Work out the finished part from the listing and answer in its coordinate system (mm). Face numbers are marked on the shaded views. Give positions to 0.01 mm unless a question says otherwise; leave off trailing zeros. Order: outer loops, then holes, each group sorted by start corner. A loop starts at its lowest first (then second) coordinate and runs counter-clockwise, first axis right, second up. Notation, with made-up numbers: (23, 86) -> (68, 86) arc R7 ccw to (68, 98) -> close; hole circle Ø7 at (28, -23). An arc over 180 degrees is marked (long way). Use a Markdown table: item, result. Add a question column.
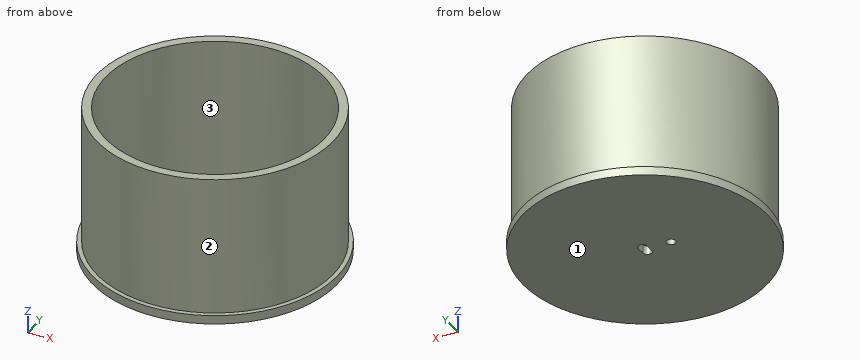
```python
from build123d import *

# Parameters (mm, degrees)
SKETCH1_R           = 88.9
BOSS_EXTRUDE1_DEPTH = 6.35
SKETCH2_R           = 3.302
CUT_EXTRUDE1_DEPTH  = 126.88384527
SKETCH3_R           = 85.725
SKETCH3_R_2         = 79.375
BOSS_EXTRUDE2_DEPTH = 101.6


with BuildPart() as part:
    # Sketch1 → Boss-Extrude1 (new body)
    with BuildSketch(Plane.XY):
        Circle(SKETCH1_R)
    extrude(amount=BOSS_EXTRUDE1_DEPTH)

    # Sketch2 → Cut-Extrude1 (cut, through all)
    with BuildSketch(Plane(origin=(0, 0, 0), x_dir=(-1, 0, 0), z_dir=(0, 0, -1))):
        with Locations((19.05, 0)):
            Circle(SKETCH2_R)
        with BuildLine():
            Line((3.081986422, 3.266652236), (3.265367316, -3.083347764))
            ThreePointArc((3.265367316, -3.083347764), (0.183342684, -6.348676869), (-3.081986422, -3.266652236))
            Line((-3.081986422, -3.266652236), (-3.265367316, 3.083347764))
            ThreePointArc((-3.265367316, 3.083347764), (-0.183342684, 6.348676869), (3.081986422, 3.266652236))
        make_face()
    extrude(amount=-CUT_EXTRUDE1_DEPTH, mode=Mode.SUBTRACT)

    # Sketch3 → Boss-Extrude2 (add)
    with BuildSketch(Plane.XY.offset(6.35)):
        Circle(SKETCH3_R)
        Circle(SKETCH3_R_2, mode=Mode.SUBTRACT)
    extrude(amount=BOSS_EXTRUDE2_DEPTH)


solid = part.part
```
1) Flat-ended cylindrical pins translate along their axes: pin 1 (10 mm diameter, centred on y = -69, z = 66.5, fed in from +X); pin 2 (1 mm diameter, centred on y = -68.5, z = 67, fed in from +X); pin 3 (10.5 mm diameter, centred on x = -19.05, y = 0, fed in from +Z). Find the tip coordinate at first contact, or state that the pin passes through.
2) The part is cut by section B-B, the plane y = 0. Determine the outline of the cut face in (x, z) (3 decimals).
3) The part is cut by section D-D, the plane y = 49. Determine the outline of the cut face in (x, z), then the cut area to 3 significant figures.
4) The part is cut by section C-C, the plane z = 86. Determine the outline of the cut face in (x, y) (3 decimals).
5) Determine the mould class of the marked faces 1, 2 and 3 for opening direction X: released by +X, released by -X, zero draft, split by the parting line, or undercut.
6) The part is cut by section A-A, the plane x = 0. Determine the outline of the cut face in (y, z) (3 decimals).
7) Straight lines are drawn through the part: line 1 (Y direction, x = 0, z = 27) (3 decimals); line 2 (Z direction, x = 72.5, y = -21); line 3 (X direction, y = 36.5, z = 52). For each, find the intervals that lie inside material, in ascending order.
A:
| question | item | result |
|---|---|---|
| 1 | pin 1 | x = 57.03 |
| 1 | pin 2 | x = 52.2 |
| 1 | pin 3 | z = 6.35 |
| 2 | outline | (-88.9, 0) -> (-22.352, 0) -> (-22.352, 6.35) -> (-79.375, 6.35) -> (-79.375, 107.95) -> (-85.725, 107.95) -> (-85.725, 6.35) -> (-88.9, 6.35) -> close; (-15.748, 0) -> (-3.176, 0) -> (-3.176, 6.35) -> (-15.748, 6.35) -> close; (3.176, 0) -> (88.9, 0) -> (88.9, 6.35) -> (85.725, 6.35) -> (85.725, 107.95) -> (79.375, 107.95) -> (79.375, 6.35) -> (3.176, 6.35) -> close |
| 3 | outline | (-74.18, 0) -> (74.18, 0) -> (74.18, 6.35) -> (70.34, 6.35) -> (70.34, 107.95) -> (62.45, 107.95) -> (62.45, 6.35) -> (-62.45, 6.35) -> (-62.45, 107.95) -> (-70.34, 107.95) -> (-70.34, 6.35) -> (-74.18, 6.35) -> close |
| 3 | area | 2,550 mm^2 |
| 4 | outline | circle Ø171.45 at (0, 0); hole circle Ø158.75 at (0, 0) |
| 5 | face 1 | zero draft |
| 5 | face 2 | split by the parting line |
| 5 | face 3 | undercut |
| 6 | outline | (-88.9, 0) -> (-6.349, 0) -> (-6.349, 6.35) -> (-79.375, 6.35) -> (-79.375, 107.95) -> (-85.725, 107.95) -> (-85.725, 6.35) -> (-88.9, 6.35) -> close; (6.349, 0) -> (88.9, 0) -> (88.9, 6.35) -> (85.725, 6.35) -> (85.725, 107.95) -> (79.375, 107.95) -> (79.375, 6.35) -> (6.349, 6.35) -> close |
| 7 | line 1 | -85.725 to -79.375, 79.375 to 85.725 |
| 7 | line 2 | 0 to 6.35 |
| 7 | line 3 | -77.57 to -70.49, 70.49 to 77.57 |
